```python
from build123d import *

# Parameters (mm, degrees)
SKETCH2_W          = 2.233127964
SKETCH2_H          = 31.607349632
CUT_EXTRUDE1_DEPTH = 80


with BuildPart() as part:
    # Sketch1 → Revolve1 (revolve)
    with BuildSketch(Plane.XY, mode=Mode.PRIVATE) as revolve1_sk:
        Polygon((0, 0), (0, 30), (10, 30), (10, 5), (70, 5), (70, 15), (80, 15), (80, 0), align=None)
    revolve(revolve1_sk.sketch.rotate(Axis((80, 0, 0), (-1, 0, 0)), 90), axis=Axis((80, 0, 0), (-1, 0, 0)))

    # Sketch2 → Cut-Extrude1 (cut)
    with BuildSketch(Plane(origin=(80, 0, 0), x_dir=(0, 0, -1), z_dir=(1, 0, 0))):
        with Locations((0, 15.803674816)):
            Rectangle(SKETCH2_W, SKETCH2_H)
    extrude(amount=-CUT_EXTRUDE1_DEPTH, mode=Mode.SUBTRACT)


solid = part.part
```
Source: CAD feature listing. Evaluate the final solid. Frame: model axes, mm. A direction names the side the tool comes from. Coordinates: 2 decimals unless noted, no trailing zeros. Loops run counter-clockwise (first coordinate to the right, second up) from the corner with the lowest first, then second, coordinate; pieces in that order, holes last. Notation, with made-up numbers: M 85.5,-6.5 L 129.5,-6.5 A30 ccw 129.5,23.5 Z; hole C 72.5,73.5 d7. An arc over 180 degrees is marked long. Use a Markdown table: item, result. Add a question column.
Q1. Draft query along X for faces 4 (the flat face through (34, 4, 1.117)), 5 (the flat face through (80, -0.2, 0.2)), 6 (the flat face through (10, 0, -6)). Return one class per face: pulls with the +X half, pulls with the -X half, needs draft (parallel to the pull), parting line crosses it, or undercut.
Q2. First-contact query: pin 1 (10 mm diameter, centred on x = 55, y = 6.5, fed in from -Z); pin 2 (1.8 mm diameter, centred on x = 29.5, z = -0.5, fed in from +Y); pin 3 (12 mm diameter, centred on x = 14.5, y = -23, fed in from +Z). Flat tips, straight axial feed; report the tip coordinate or a pass-through.
Q3. Section query D-D, the plane z = 0. Return loops of the section in (x, y).
Q4. Section query B-B, the plane y = 7.5. Return loops of the section in (x, z).
Q5. Section query A-A, the plane z = 12. Return loops of the section in (x, y), and give its area (3 significant figures).
Q6. Access query for faces 1 (the flat face through (41, 0, 0)), 2 (the flat face through (0, -0.4, -0.4)), 3 (the cylindrical face through (40, -5, 0)). Directions: +Z, -Z, +X, -X, +Y, -Y. A direction counts if a zero-diameter tool reaches every point of the face in a straight line with its end or side. Return the directions, or none.
Q7. Material intervals for L1, parallel to X at y = -5.5, z = -8; L2, parallel to X at y = 18.5, z = -23.5; L3, parallel to Y at x = 8, z = -0.5, sorted ascending.
Result:
| question | item | result |
|---|---|---|
| 1 | face 4 | needs draft |
| 1 | face 5 | pulls with the +X half |
| 1 | face 6 | undercut |
| 2 | pin 1 | stops at z = -4.77 |
| 2 | pin 2 | stops at y = 4.87 |
| 2 | pin 3 | stops at z = 23.19 |
| 3 | outline | M 0,-30 L 10,-30 L 10,-5 L 70,-5 L 70,-15 L 80,-15 L 80,0 L 0,0 Z |
| 4 | outline | M 0,-29.05 L 10,-29.05 L 10,-1.12 L 0,-1.12 Z; M 0,1.12 L 10,1.12 L 10,29.05 L 0,29.05 Z; M 70,-12.99 L 80,-12.99 L 80,-1.12 L 70,-1.12 Z; M 70,1.12 L 80,1.12 L 80,12.99 L 70,12.99 Z |
| 5 | outline | M 0,-27.5 L 10,-27.5 L 10,27.5 L 0,27.5 Z; M 70,-9 L 80,-9 L 80,9 L 70,9 Z |
| 5 | area | 730 mm2 |
| 6 | face 1 | +X, -X, +Y |
| 6 | face 2 | +Z, -Z, -X, +Y, -Y |
| 6 | face 3 | none |
| 7 | L1 | x = 0 to 10, 70 to 80 |
| 7 | L2 | x = 0 to 10 |
| 7 | L3 | y = -30 to 0 |
